Input: part model. Units: mm. Frame: model coordinates. Face numbers are marked on the shaded views. A direction names the side the tool comes from. Round coordinates to 2 decimals unless told otherwise and drop trailing zeros. Loops run counter-clockwise (first coordinate to the right, second up) from the corner with the lowest first, then second, coordinate; pieces in that order, holes last.
1) Section D-D, the plane x = 0. Return loops of the section in (y, z).
2) Section A-A, the plane z = 6. Return loops of the section in (x, y).
3) Ray query, line 1 along Y through (x, z) = (0, 1.35); line 2 along X through (y, z) = (9.5, 4.5); line 3 along Z through (x, y) = (0, 13). Return the intervals inside material, ascending.
4) Section B-B, the plane x = -16. Return loops of the section in (y, z).
5) Draft query along Z for the marked faces 1, 2 and 3. Return one class per face: pulls with the +Z half, pulls with the -Z half, needs draft (parallel to the pull), parting line crosses it, or undercut.
6) First-contact query: pin 1 (1.5 mm diameter, centred on y = -12, z = 6, fed in from +X); pin 2 (6.5 mm diameter, centred on x = 0, y = 0, fed in from -Z); pin 3 (4 mm diameter, centred on x = -13.5, z = 5.5, fed in from -Y); pin 4 (3 mm diameter, centred on x = 1, z = 5.5, fed in from -Y). Flat tips, straight axial feed; report the tip coordinate or a pass-through.
7) Section C-C, the plane y = -16. Return loops of the section in (x, z), and give its area (3 significant figures).
8) Access query for the marked faces 4, 5 and 6. Directions: +Z, -Z, +X, -X, +Y, -Y. A direction counts if a zero-diameter tool reaches every point of the face in a straight line with its end or side. Return the directions, or none.
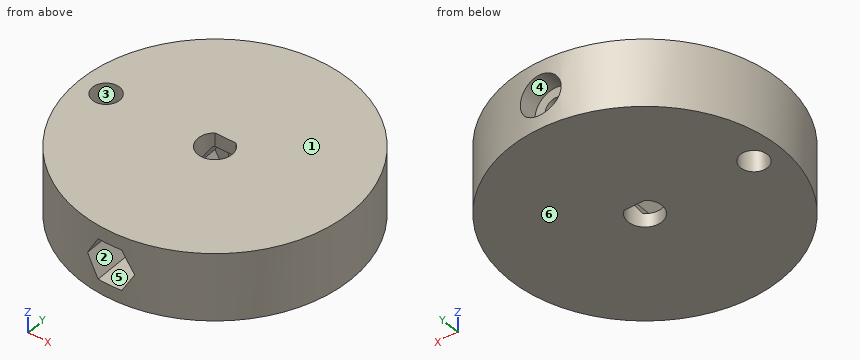
Autodesk Inventor part; units mm, degrees
ref_plane "YZ Plane" through (0, 0, 0) normal (1, 0, 0) x (0, 1, 0)
ref_plane "XZ Plane" through (0, 0, 0) normal (0, 1, 0) x (-1, 0, 0)
ref_plane "XY Plane" through (0, 0, 0) normal (0, 0, 1) x (1, 0, 0)
sketch "草圖1" plane through (0, 0, 0) normal (0, 0, 1) x (1, 0, 0)
  arc A0 (-1.5263, 1.98) -> (1.5263, 1.98) centre (0, 0) ccw
  line L0 (1.5263, 1.98) -> (-1.5263, 1.98)
  circle A1 centre (0, 0) radius 20
  point P0 (0, -2.5)
  dimension "d0" = 5
  dimension "d2" = 4.48
  dimension "d3" = 40
extrude "擠出1" add sketch "草圖1" along normal blind 10
sketch "草圖2" plane through (-1.5263, 1.98, 0) normal (0, -1, 0) x (1, 0, 0)
  line L0 (3.2584, 8) -> (4.9904, 5)
  line L1 (4.9904, 5) -> (3.2584, 2)
  line L2 (3.2584, 2) -> (-0.2057, 2)
  line L3 (-0.2057, 2) -> (-1.9378, 5)
  line L4 (-1.9378, 5) -> (-0.2057, 8)
  line L5 (-0.2057, 8) -> (3.2584, 8)
  point P0 (1.5263, 0)
  point P1 (1.5263, 5)
  point P2 (1.5263, 8)
extrude "擠出2" cut sketch "草圖2" against normal blind 2.5
extrude "擠出3" cut sketch "草圖2" along normal through all
sketch "草圖4" plane through (-1.5263, 4.48, 0) normal (0, -1, 0) x (1, 0, 0)
  circle A0 centre (1.5263, 5) radius 1.5
  circle A1 centre (1.5263, 5) radius 3
  point P0 (1.5263, 0)
  dimension "d11" = 3
  dimension "d12" = 6
extrude "擠出4" cut sketch "草圖4" against normal through all contours A0
ref_plane "工作平面1" through (-1.5263, 21.98, 0) normal (0, -1, 0) x (1, 0, 0)
sketch "草圖5" plane through (-1.5263, 21.98, 0) normal (0, -1, 0) x (1, 0, 0)
  circle A0 centre (1.5263, 5) radius 1.5
  circle A1 centre (1.5263, 5) radius 3
  point P0 (1.5263, 0)
  dimension "d16" = 6
extrude "擠出5" cut sketch "草圖5" along normal blind 5 contours A0 | A1
sketch "草圖6" plane through (0, 0, 0) normal (0, 0, -1) x (-1, 0, 0)
  circle A0 centre (16, 0) radius 2
  point P0 (0, 0)
  dimension "d19" = 4
  dimension "d20" = 16
extrude "擠出6" cut sketch "草圖6" against normal through all
properties part number "crank"
Final values:
1. outline: (-20, 0) - (-2.5, 0) - (-2.5, 2) - (-20, 2) - close; (-20, 8) - (-2.5, 8) - (-2.5, 10) - (-20, 10) - close; (1.98, 0) - (20, 0) - (20, 2) - (16.98, 2) - (16.98, 3.5) - (4.48, 3.5) - (4.48, 2) - (1.98, 2) - close; (1.98, 8) - (4.48, 8) - (4.48, 6.5) - (16.98, 6.5) - (16.98, 8) - (20, 8) - (20, 10) - (1.98, 10) - close
2. outline: (-2.89, -19.79) - (-2.89, 4.48) - (-1.12, 4.48) - (-1.12, 16.98) - (-2.83, 16.98) - (-2.83, 19.8) arc R20 ccw to start; (1.12, 4.48) - (2.89, 4.48) - (2.89, -19.79) arc R20 ccw to (2.83, 19.8) - (2.83, 16.98) - (1.12, 16.98) - close; hole circle Ø4 at (-16, 0)
3. line 1: y = -20 to -2.5, 1.98 to 20
3. line 2: x = -17.6 to -1.41, 1.41 to 17.6
3. line 3: z = 0 to 3.5, 6.5 to 10
4. outline: (-12, 0) - (-2, 0) - (-2, 10) - (-12, 10) - close; (2, 0) - (12, 0) - (12, 10) - (2, 10) - close
5. face 1: pulls with the +Z half
5. face 2: undercut
5. face 3: needs draft
6. pin 1: stops at x = 16.54
6. pin 2: stops at z = 0
6. pin 3: stops at y = -16.36
6. pin 4: stops at y = 4.48
7. outline: (-12, 0) - (12, 0) - (12, 10) - (-12, 10) - close; hole (-3.46, 5) - (-1.73, 2) - (1.73, 2) - (3.46, 5) - (1.73, 8) - (-1.73, 8) - close
7. area: 209 mm2
8. face 4: +Y
8. face 5: -Y
8. face 6: -Z, +X, -X, +Y, -Y
